For this review, take the finished solid that the model builds, in its own axes (mm). A direction names the side the tool comes from. Coordinates: 2 decimals unless noted, no trailing zeros. Loops run counter-clockwise (first coordinate to the right, second up) from the corner with the lowest first, then second, coordinate; pieces in that order, holes last. Notation, with made-up numbers: M -12.75,57 L 46.25,57 A23 ccw 46.25,76 Z; hole C 79.5,22.25 d11. An arc over 180 degrees is marked long. Write item = value, one per line.
Autodesk Inventor part; units mm, degrees
ref_plane "YZ Plane" through (0, 0, 0) normal (1, 0, 0) x (0, 1, 0)
ref_plane "XZ Plane" through (0, 0, 0) normal (0, 1, 0) x (-1, 0, 0)
ref_plane "XY Plane" through (0, 0, 0) normal (0, 0, 1) x (1, 0, 0)
sketch "Sketch4" plane through (0, 0, 0) normal (0, 0, 1) x (1, 0, 0)
  line L0 (-144.3789, 43.7906) -> (-144.3789, -108.6094)
  line L1 (-144.3789, -108.6094) -> (160.4211, -108.6094)
  line L2 (160.4211, -108.6094) -> (160.4211, -7.0094)
  line L3 (160.4211, -7.0094) -> (-144.3789, 43.7906)
  point P0 (0, 0)
  dimension "d6" = 304.8
  dimension "d7" = 152.4
  dimension "d8" = 101.6
extrude "Body" add sketch "Sketch4" along normal blind 1371.6
sketch "Sketch5" plane through (160.4211, -108.6094, 0) normal (1, 0, 0) x (0, 0, -1)
  line L0 (-1371.6, 0) -> (-1371.6, 101.6)
  line L1 (0, 0) -> (-1371.6, 0)
  line L2 (-1371.6, 0) -> (-1318.7374, 299.7986)
  line L3 (-1318.7374, 299.7986) -> (-1508.9577, 299.7986)
  line L4 (-1371.6, 152.4) -> (-1371.6, 0)
  line L5 (-1508.9577, 299.7986) -> (-1371.6, 0)
  point P0 (0, 108.6094)
  dimension "d11" = 10
extrude "LeftBevel" cut sketch "Sketch5" against normal blind 1371.6
sketch "Sketch6" plane through (160.4211, -108.6094, 0) normal (1, 0, 0) x (0, 0, -1)
  line L0 (0, 0) -> (0, 101.6)
  line L1 (0, 0) -> (-1371.6, 0)
  line L2 (0, 0) -> (-29.2918, 166.1219)
  line L3 (-29.2918, 166.1219) -> (35.444, 166.1219)
  line L4 (35.444, 166.1219) -> (0, 0)
  point P0 (0, 108.6094)
  dimension "d14" = 10
extrude "RightBevel" cut sketch "Sketch6" against normal blind 1371.6
sketch "Sketch7" plane through (0, 0, 1371.6) normal (0, 0, 1) x (1, 0, 0)
  line L0 (-144.3789, 43.7906) -> (-144.3789, -108.6094)
  line L1 (-144.3789, -108.6094) -> (-110.1629, 85.4397)
  line L2 (-110.1629, 85.4397) -> (-236.272, 85.4397)
  line L3 (-236.272, 85.4397) -> (-144.3789, -108.6094)
  point P0 (0, 0)
  dimension "d17" = 10
extrude "BackBevel" cut sketch "Sketch7" against normal blind 1371.6
sketch "Sketch8" plane through (0, 0, 1371.6) normal (0, 0, 1) x (1, 0, 0)
  line L0 (160.4211, -108.6094) -> (160.4211, -7.0094)
  line L1 (-144.3789, -108.6094) -> (160.4211, -108.6094)
  line L2 (160.4211, -108.6094) -> (129.3641, 67.5233)
  line L3 (129.3641, 67.5233) -> (267.9679, 67.5233)
  line L4 (267.9679, 67.5233) -> (160.4211, -108.6094)
  point P0 (0, 0)
  dimension "d20" = 10
extrude "FrontBevel" cut sketch "Sketch8" against normal blind 1371.6
sketch "Sketch9" plane through (-144.3789, -108.6094, 0) normal (0, -1, 0) x (1, 0, 0)
  line L0 (286.893, 1320.8) -> (58.293, 1320.8)
  line L1 (58.293, 1320.8) -> (58.293, 50.8)
  line L2 (58.293, 50.8) -> (286.893, 50.8)
  line L3 (286.893, 50.8) -> (286.893, 1320.8)
  line L4 (304.8, 0) -> (304.8, 1371.6)
  line L5 (0, 0) -> (304.8, 0)
  line L6 (0, 1371.6) -> (304.8, 1371.6)
  point P0 (144.3789, 0)
  dimension "d24" = 228.6
  dimension "d25" = 17.907
  dimension "d26" = 50.8
  dimension "d31" = 50.8
extrude "BottomEx" add sketch "Sketch9" against normal blind 152.4
sketch "Sketch10" plane through (-144.3789, 43.7906, 0) normal (0, 1, 0) x (1, 0, 0)
  line L0 (58.293, -1320.8) -> (286.893, -1320.8)
  line L1 (286.893, -1320.8) -> (286.893, -50.8)
  line L2 (286.893, -50.8) -> (58.293, -50.8)
  line L3 (58.293, -50.8) -> (58.293, -1320.8)
  line L4 (58.293, -50.8) -> (286.893, -50.8)
  line L5 (286.893, -50.8) -> (58.293, -50.8)
  line L6 (58.293, -50.8) -> (58.293, -1320.8)
  line L7 (58.293, -1320.8) -> (286.893, -1320.8)
  line L8 (286.893, -1320.8) -> (286.893, -50.8)
  point P0 (144.3789, 0)
  point P1 (26.1051, -50.8)
extrude "Extrusion8" cut sketch "Sketch10" against normal blind 57.15
sketch "Sketch11" plane through (-144.3789, -13.3594, 0) normal (0, 1, 0) x (1, 0, 0)
  line L0 (70.993, -266.7) -> (274.193, -266.7)
  line L1 (274.193, -266.7) -> (274.193, -63.5)
  line L2 (274.193, -63.5) -> (70.993, -63.5)
  line L3 (70.993, -63.5) -> (70.993, -266.7)
  line L4 (58.293, -1320.8) -> (58.293, -50.8)
  line L5 (58.293, -50.8) -> (286.893, -50.8)
  point P0 (144.3789, 0)
  dimension "d32" = 203.2
  dimension "d33" = 203.2
  dimension "d34" = 12.7
  dimension "d35" = 12.7
extrude "Extrusion9" cut sketch "Sketch11" against normal blind 174.625
sketch "Sketch12" plane through (-144.3789, -13.3594, 0) normal (0, 1, 0) x (1, 0, 0)
  line L0 (58.293, -1320.8) -> (58.293, -50.8)
  line L1 (286.893, -1320.8) -> (58.293, -1320.8)
  line L2 (70.993, -1308.1) -> (274.193, -1308.1)
  line L3 (274.193, -1308.1) -> (274.193, -1104.9)
  line L4 (274.193, -1104.9) -> (70.993, -1104.9)
  line L5 (70.993, -1104.9) -> (70.993, -1308.1)
  point P0 (144.3789, 0)
  dimension "d38" = 203.2
  dimension "d39" = 203.2
  dimension "d40" = 12.7
  dimension "d41" = 12.7
extrude "Extrusion10" cut sketch "Sketch12" against normal blind 166.6875
sketch "Sketch13" plane through (-144.3789, -13.3594, 0) normal (0, 1, 0) x (1, 0, 0)
  line L0 (70.993, -266.7) -> (70.993, -63.5)
  line L1 (70.993, -266.7) -> (274.193, -266.7)
  line L2 (274.193, -266.7) -> (70.993, -266.7)
  line L3 (274.193, -266.7) -> (70.993, -266.7)
  line L4 (70.993, -317.5) -> (274.193, -317.5)
  line L5 (274.193, -317.5) -> (274.193, -520.7)
  line L6 (274.193, -520.7) -> (70.993, -520.7)
  line L7 (70.993, -520.7) -> (70.993, -317.5)
  point P0 (144.3789, 0)
  dimension "d44" = 0
  dimension "d45" = 50.8
  dimension "d46" = 203.2
  dimension "d47" = 203.2
extrude "Extrusion11" cut sketch "Sketch13" against normal blind 166.6875
sketch "Sketch14" plane through (-144.3789, -13.3594, 0) normal (0, 1, 0) x (1, 0, 0)
  line L0 (70.993, -1308.1) -> (70.993, -1104.9)
  line L1 (70.993, -1104.9) -> (274.193, -1104.9)
  line L2 (70.993, -1054.1) -> (274.193, -1054.1)
  line L3 (274.193, -1054.1) -> (274.193, -850.9)
  line L4 (274.193, -850.9) -> (70.993, -850.9)
  line L5 (70.993, -850.9) -> (70.993, -1054.1)
  point P0 (144.3789, 0)
  dimension "d50" = 0
  dimension "d51" = 50.8
  dimension "d52" = 203.2
  dimension "d53" = 203.2
extrude "Extrusion12" cut sketch "Sketch14" against normal blind 166.6875
sketch "Sketch15" plane through (-144.3789, -13.3594, 0) normal (0, 1, 0) x (1, 0, 0)
  line L0 (70.993, -825.5) -> (274.193, -825.5)
  line L1 (274.193, -825.5) -> (274.193, -546.1)
  line L2 (274.193, -546.1) -> (70.993, -546.1)
  line L3 (70.993, -546.1) -> (70.993, -825.5)
  line L4 (70.993, -520.7) -> (70.993, -317.5)
  line L5 (274.193, -520.7) -> (70.993, -520.7)
  line L6 (70.993, -850.9) -> (274.193, -850.9)
  point P0 (144.3789, 0)
  dimension "d56" = 279.4
  dimension "d57" = 203.2
  dimension "d58" = 0
  dimension "d59" = 25.4
  dimension "d60" = 25.4
extrude "Extrusion13" cut sketch "Sketch15" against normal blind 166.6875
sketch "Sketch16" plane through (-144.3789, -108.6094, 0) normal (-0.9848, 0.1736, 0) x (0, 0, 1)
  line L0 (297.688, 126.8744) -> (1073.912, 126.8744)
  line L1 (1073.912, 126.8744) -> (1073.912, 29.8464)
  line L2 (1073.912, 29.8464) -> (297.688, 29.8464)
  line L3 (297.688, 29.8464) -> (297.688, 126.8744)
  line L4 (0, 0) -> (0, 150.3331)
  point P0 (0, 132.0305)
  dimension "d63" = 97.028
  dimension "d64" = 776.224
  dimension "d65" = 297.688
extrude "Extrusion14" cut sketch "Sketch16" against normal blind 15.24
properties part number "FullConsole"
Q1. For line 1 along Z through (x, y) = (-16, -74.5); line 2 along Z through (x, y) = (-33.5, 6.5); line 3 along X through (y, z) = (7.5, 650), list the stretches that pass through material, from the lowest coordinate up.
Solved:
line_1 = 6.01 to 63.5, 266.7 to 317.5, 520.7 to 546.1, 825.5 to 850.9, 1054.1 to 1104.9, 1308.1 to 1365.59
line_2 = 20.3 to 50.8, 1320.8 to 1351.3
line_3 = -108.43 to -86.09
Q2. Add section A-A (z = 720). Write out the cut boundary in (x, y).
Solved:
outline = M -144.38,-108.61 L -73.39,-108.61 L -73.39,-13.36 L -86.09,-13.36 L -86.09,34.08 L -118.27,39.44 L -122.35,16.34 L -107.34,13.69 L -124.19,-81.86 L -139.2,-79.22 Z; M 129.81,-108.61 L 160.42,-108.61 L 142.51,-7.05 L 142.51,-13.36 L 129.81,-13.36 Z
Q3. For pin 1 Ø6 at (x, y) = (-18.5, -91.5) entering from -Z; pin 2 Ø8 at (x, y) = (-16.5, 21) entering from -Z; pin 3 Ø8 at (x, y) = (-48.5, -25.5) entering from -Z, all flat-tipped, find the tip position at first contact; note any pin that passes through.
Solved:
pin_1 = 2.49
pin_2 = 22.15
pin_3 = 13.95
Q4. Machinability: for faces 5 (the face through (-73.386, -60, 684)), 6 (the face through (-140.21, -84.97, 695.4)), which of the approach directions +Z, -Z, +X, -X, +Y, -Y give a long, thin tool a straight path to every point of the face, cutting with its end or side? Answer none if there is none.
Solved:
face_5 = +Y, -Y
face_6 = +Z, -Z, -X, +Y
Q5. Add section C-C (y = -95). Write out the cut boundary in (x, z).
Solved:
outline = M -141.98,2.4 L 158.02,2.4 L 158.02,1369.2 L -141.98,1369.2 Z; hole M -73.39,63.5 L 129.81,63.5 L 129.81,266.7 L -73.39,266.7 Z; hole M -73.39,317.5 L 129.81,317.5 L 129.81,520.7 L -73.39,520.7 Z; hole M -73.39,546.1 L 129.81,546.1 L 129.81,825.5 L -73.39,825.5 Z; hole M -73.39,850.9 L 129.81,850.9 L 129.81,1054.1 L -73.39,1054.1 Z; hole M -73.39,1104.9 L 129.81,1104.9 L 129.81,1308.1 L -73.39,1308.1 Z
Q6. Draft analysis for pull direction Z (two halves, no side actions). For faces 1 (the face through (129.814, -60, 954)), 2 (the face through (-93.571, 35.323, 682.686)), 3 (the face through (30, -60, 1104.9)), 4 (the face through (10.15, -52.07, 9.97)), state which applies: +Z half, -Z half, draft (parallel to the pull), parting line (faces both ways), or undercut.
Solved:
face_1 = undercut
face_2 = draft
face_3 = undercut
face_4 = -Z half
Q7. Add section B-B (x = -18). Write out the cut boundary in (y, z).
Solved:
outline = M -108.61,0 L 22.73,23.16 L 22.73,50.8 L -13.36,50.8 L -13.36,63.5 L -108.61,63.5 Z; M -108.61,266.7 L -13.36,266.7 L -13.36,317.5 L -108.61,317.5 Z; M -108.61,520.7 L -13.36,520.7 L -13.36,546.1 L -108.61,546.1 Z; M -108.61,825.5 L -13.36,825.5 L -13.36,850.9 L -108.61,850.9 Z; M -108.61,1054.1 L -13.36,1054.1 L -13.36,1104.9 L -108.61,1104.9 Z; M -108.61,1308.1 L -13.36,1308.1 L -13.36,1320.8 L 22.73,1320.8 L 22.73,1348.44 L -108.61,1371.6 Z
Q8. Add section D-D (x = 107). Write out the cut boundary in (y, z).
Solved:
outline = M -108.61,0 L 1.89,19.48 L 1.89,50.8 L -13.36,50.8 L -13.36,63.5 L -108.61,63.5 Z; M -108.61,266.7 L -13.36,266.7 L -13.36,317.5 L -108.61,317.5 Z; M -108.61,520.7 L -13.36,520.7 L -13.36,546.1 L -108.61,546.1 Z; M -108.61,825.5 L -13.36,825.5 L -13.36,850.9 L -108.61,850.9 Z; M -108.61,1054.1 L -13.36,1054.1 L -13.36,1104.9 L -108.61,1104.9 Z; M -108.61,1308.1 L -13.36,1308.1 L -13.36,1320.8 L 1.89,1320.8 L 1.89,1352.12 L -108.61,1371.6 Z
